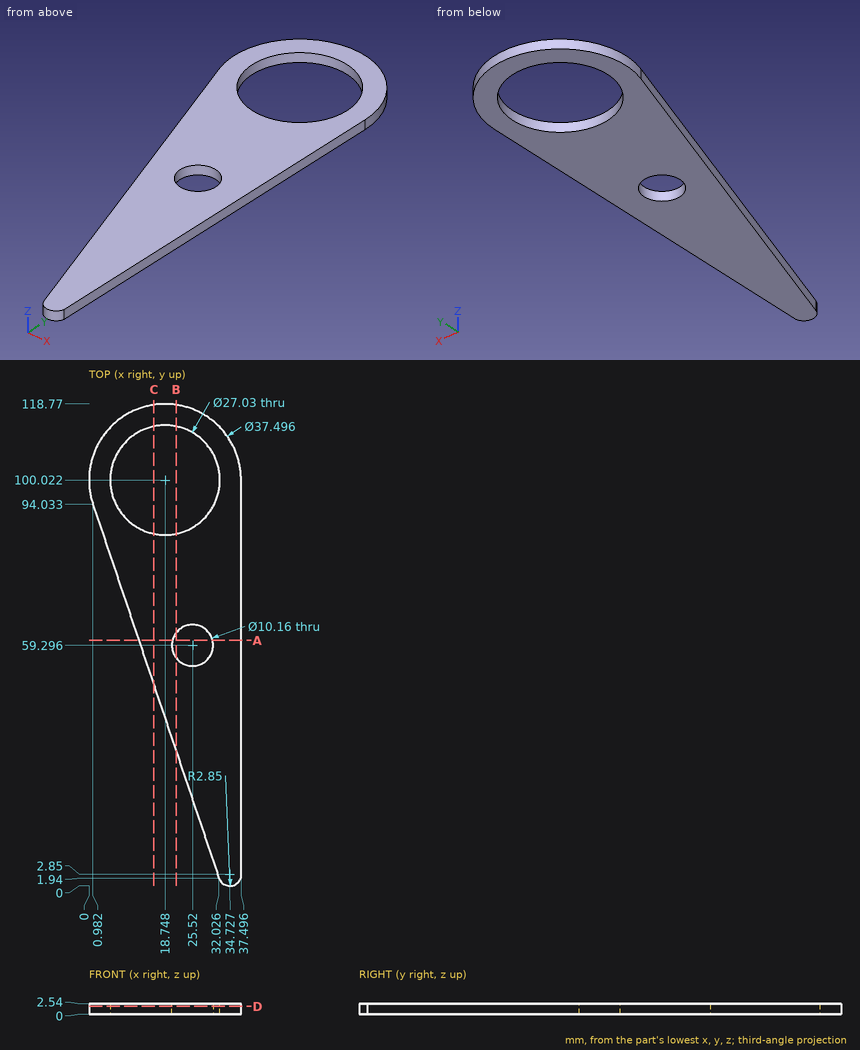
Verification items for this drawing (mm, ordinates from the low corner). Coordinates: 2 decimals unless noted, no trailing zeros. Order: outer loops, then holes, each group sorted by start corner. A loop starts at its lowest first (then second) coordinate and runs counter-clockwise, first axis right, second up. Notation, with made-up numbers: (86.25, -28) -> (124.25, -28) arc R24 ccw to (124.25, 7) -> close; hole circle Ø9 at (78.25, 21.5). An arc over 180 degrees is marked (long way). Answer as CSV lines item,"result". Start each with the question number.
1) Cross-section at D-D, the plane z = 1.95. Give the number of separate pieces and of enclosed holes in the cut face, then the cut area to 3 significant figures.
2) Material ranges on L1, parallel to X at y = 99.5, z = 1.25; L2, parallel to X at y = 105.5, z = 2.2; L3, parallel to X at y = 82.5, z = 2.3 (1 decimal), recorded low to high. Write a range as [from, to].
3) Cross-section at C-C, the plane x = 16. Record the boundary of the cut face in (y, z) (1 decimal), then the cut area to 3 significant figures.
4) Cross-section at B-B, the plane x = 21.5. Record the boundary of the cut face in (y, z).
5) Gauge pin test, flat end, axial feed: pin 1 Ø5 at (x, y) = (26, 63.5) entering from -Z. Record the tip position at first contact, or that the pin passes through.
6) Cross-section at A-A, the plane y = 60.5. Record the boundary of the cut face in (x, z) (1 decimal).
Conclusion:
1,separate pieces,"1"
1,enclosed holes,"2"
1,area,"2,060 mm²"
2,L1,"x = [0.01, 5.24], [32.25, 37.5]"
2,L2,"x = [0.82, 6.39], [31.1, 36.68]"
2,L3,"x = [4.9, 37.5]"
3,outline,"(49.5, 0) -> (86.8, 0) -> (86.8, 2.5) -> (49.5, 2.5) -> close; (113.3, 0) -> (118.6, 0) -> (118.6, 2.5) -> (113.3, 2.5) -> close"
3,area,"108 mm²"
4,outline,"(33.17, 0) -> (56.19, 0) -> (56.19, 2.54) -> (33.17, 2.54) -> close; (62.4, 0) -> (86.79, 0) -> (86.79, 2.54) -> (62.4, 2.54) -> close; (113.25, 0) -> (118.57, 0) -> (118.57, 2.54) -> (113.25, 2.54) -> close"
5,pin 1,"stops at z = 0"
6,outline,"(12.3, 0) -> (20.6, 0) -> (20.6, 2.5) -> (12.3, 2.5) -> close; (30.5, 0) -> (37.5, 0) -> (37.5, 2.5) -> (30.5, 2.5) -> close"
